Geometry: final body of the model. Coordinates: model frame, mm. A direction names the side the tool comes from. Round coordinates to 2 decimals unless told otherwise and drop trailing zeros. Loops run counter-clockwise (first coordinate to the right, second up) from the corner with the lowest first, then second, coordinate; pieces in that order, holes last. Notation, with made-up numbers: (68.25, -24) - (107.25, -24) arc R26 cw to (107.25, -2) - close; hole circle Ø2 at (55, 65.25). An arc over 180 degrees is marked (long way). Answer in a Markdown table with one row per item. Add a question column.
from build123d import *

# Parameters (mm, degrees)
F1_DEPTH = 101.6
F3_DEPTH = 6.35
F4_R     = 6.35
F5_DEPTH = 25.4
F6_R     = 6.35
F7_DEPTH = 6.35


with BuildPart() as f1:
    # F0 (on Front) → F1 (new body)
    with BuildSketch(Plane.XZ):
        Polygon((-25.4, 0), (0, 0), (0, 12.7), (-25.4, 12.7), (-254, 32.699908482), (-254, 19.999908482), align=None)
    extrude(amount=F1_DEPTH)

    # F2 (on face) → F3 (join)
    with BuildSketch(Plane(origin=(0.9097243914, 0, 10.3981973753), x_dir=(0.9961946981, 0, -0.0871557427), z_dir=(0.0871557427, 0, 0.9961946981))):
        Polygon((-26.4102232644, 0), (-255.8834381268, 0), (-26.4102232644, -41.275), align=None)
        Polygon((-26.4102232644, -60.325), (-255.8834381268, -101.6), (-26.4102232644, -101.6), align=None)
    extrude(amount=F3_DEPTH)

    # F4 (on Top) → F5 (cut)
    with BuildSketch(Plane.XY):
        with Locations((-228.6, -25.4)):
            Circle(F4_R)
        with Locations((-228.6, -76.2)):
            Circle(F4_R)
    extrude(amount=F5_DEPTH, mode=Mode.SUBTRACT)

    # F6 (on face) → F7 (cut)
    with BuildSketch(Plane(origin=(0, 0, 0), x_dir=(1, 0, 0), z_dir=(0, 0, -1))):
        with Locations((-12.7, 25.4)):
            Circle(F6_R)
        with Locations((-12.7, 76.2)):
            Circle(F6_R)
    extrude(amount=-F7_DEPTH, mode=Mode.SUBTRACT)


solid = f1.part
1) Reachability of faces 1 (the flat face through (-254, -50, 26)), 2 (the flat face through (-25.127, -81.251, 15.819)), 3 (the flat face through (-163.5, -50.089, 24.782)), 4 (the flat face through (-13, -76, 6.35)), 5 (the flat face through (-89.95, -89.85, 24.72)) from +Z, -Z, +X, -X, +Y, -Y: full face, straight path, thin tool, end or side. Return the list, or none.
2) Section B-B, the plane x = -40.5. Return the cut outline in (y, z).
3) Pull-direction query (Z, two-part tool) for faces 6 (the flat face through (-13, -50, 0)), 7 (the cylindrical face through (-222.543, -74.293, 21.254)), 8 (the flat face through (-25.127, -20.926, 15.819)); classes: pulls with the +Z half, pulls with the -Z half, needs draft (parallel to the pull), parting line crosses it, or undercut.
4) Section D-D, the plane x = -12.7. Return the cut outline in (y, z).
5) Contact query for flat-ended pins moving along their axis: pin 1 Ø1.5 at (x, y) = (-191.5, -32) entering from +Z; pin 2 Ø1 at (x, y) = (-137.5, -48) entering from -Z; pin 3 Ø10 at (x, y) = (-13, -75.5) entering from -Z. Output: stop coordinate, or through.
6) Material intervals for line 1 along Y through (x, z) = (-12.7, 1.75); line 2 along Y through (x, z) = (-226, 24); line 3 along Y through (x, z) = (-150.5, 26.5), sorted ascending. Write a range as from..to.
7) Section A-A, the plane z = 36.5. Return the cut outline in (x, y), and give its area (3 significant figures).
8) Section C-C, the plane y = -37.5. Return the cut outline in (x, z), and give its area (3 significant figures).
Evaluation:
| question | item | result |
|---|---|---|
| 1 | face 1 | +Z, -Z, -X, +Y, -Y |
| 1 | face 2 | +X, +Y, -Y |
| 1 | face 3 | +Z |
| 1 | face 4 | -Z |
| 1 | face 5 | +Z, +X, +Y, -Y |
| 2 | outline | (-101.6, 1.32) - (0, 1.32) - (0, 20.4) - (-38.45, 20.4) - (-38.55, 14.02) - (-63.05, 14.02) - (-63.15, 20.4) - (-101.6, 20.4) - close |
| 3 | face 6 | pulls with the -Z half |
| 3 | face 7 | needs draft |
| 3 | face 8 | undercut |
| 4 | outline | (-101.6, 0) - (-82.55, 0) - (-82.55, 6.35) - (-69.85, 6.35) - (-69.85, 0) - (-31.75, 0) - (-31.75, 6.35) - (-19.05, 6.35) - (-19.05, 0) - (0, 0) - (0, 12.7) - (-101.6, 12.7) - close |
| 5 | pin 1 | stops at z = 27.3 |
| 5 | pin 2 | stops at z = 9.76 |
| 5 | pin 3 | stops at z = 6.35 |
| 6 | line 1 | y = -101.6..-82.55, -69.85..-31.75, -19.05..0 |
| 6 | line 2 | y = -101.6..-81.99, -70.41..-31.19, -19.61..0 |
| 6 | line 3 | y = -101.6..-82.96, -18.64..0 |
| 7 | outline | (-253.67, -101.6) - (-224.58, -101.6) - (-224.58, -96.39) - close; (-253.67, 0) - (-224.58, -5.21) - (-224.58, 0) - close |
| 7 | area | 152 mm² |
| 8 | outline | (-254, 20) - (-25.4, 0) - (0, 0) - (0, 12.7) - (-25.4, 12.7) - (-24.85, 19.03) - (-45.75, 20.86) - (-46.31, 14.53) - (-254, 32.7) - close |
| 8 | area | 3,360 mm² |
